```python
from build123d import *

# Parameters (mm, degrees)
BOSS_EXTRU_1_DEPTH      = 2
ESQUISSE2_R             = 1.5
ENL_V_MAT_EXTRU_1_DEPTH = 2


with BuildPart() as part:
    # Esquisse1 → Boss.-Extru.1 (new body)
    with BuildSketch(Plane.XY):
        with BuildLine():
            Line((-36.939711753, -10.835982903), (-28.105322833, -36.349774711))
            ThreePointArc((-28.105322833, -36.349774711), (-25.588682721, -38.027012465), (-23.297783694, -36.052579486))
            Line((-23.297783694, -36.052579486), (-18.763886374, -14.728100955))
            ThreePointArc((-18.763886374, -14.728100955), (-18.961021654, -12.824866099), (-20.44620762, -11.61847152))
            Line((-20.44620762, -11.61847152), (-33.863669528, -7.622008589))
            ThreePointArc((-33.863669528, -7.622008589), (-36.383421268, -8.289397427), (-36.939711753, -10.835982903))
        make_face()
        Polygon((-24.085912758, -15.751447914), (-26.31791891, -26.23061998), (-30.620361937, -13.805127209), align=None, mode=Mode.SUBTRACT)
    extrude(amount=-BOSS_EXTRU_1_DEPTH)

    # Esquisse2 → Enlèv. mat.-Extru.1 (cut)
    with BuildSketch(Plane.XY):
        with Locations((-34.577323623, -10.017983929)):
            Circle(ESQUISSE2_R)
        with Locations((-21.159861715, -14.01444686)):
            Circle(ESQUISSE2_R)
    extrude(amount=-ENL_V_MAT_EXTRU_1_DEPTH, mode=Mode.SUBTRACT)


solid = part.part
```
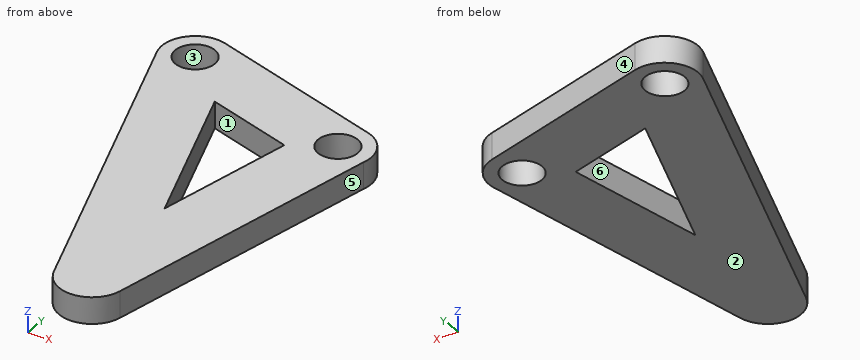
Verification items for the finished model (mm, model axes). Face numbers are marked on the shaded views. A direction names the side the tool comes from. Round coordinates to 2 decimals unless told otherwise and drop trailing zeros. Order: outer loops, then holes, each group sorted by start corner. A loop starts at its lowest first (then second) coordinate and runs counter-clockwise, first axis right, second up. Notation, with made-up numbers: (-14, -17.5) -> (9, -17.5) arc R14 ccw to (9, 6.5) -> close; hole circle Ø4 at (82.25, 47.5). An arc over 180 degrees is marked (long way). Put each result on its own line as item: value. Start each with the question number.
(1) Tool access check on the marked faces 5 and 6. Record the directions out of +Z, -Z, +X, -X, +Y, -Y that give a thin tool (end or side, any length) a straight path to the whole face; none if there is none.
(2) Section check B-B (y = -23). Enter the section's corners in (x, z), then the cut area to 3 significant figures.
(3) Draft check along Y on the marked faces 1, 2, 3 and 4. Enter one of: +Y half, -Y half, draft (parallel to the pull), parting line (faces both ways), or undercut.
(4) Section check C-C (z = -0.75). Enter the section's corners in (x, y).
(5) Section check D-D (x = -31.25). Enter the section's corners in (y, z).
(6) Section check A-A (x = -20). Enter the section's corners in (y, z), then the cut area to 3 significant figures.
(7) Depth check by flat-ended pin: pin 1 Ø1 at (y, z) = (-34, -1.5) entering from +X. Enter the tip coordinate at first touch or a pass-through.
(8) Material ranges on line 1 along X through (y, z) = (-19, -0.9); line 2 along X through (y, z) = (-25, -0.8); line 3 along X through (y, z) = (-28.5, -0.3), recorded low to high.
Completed:
1. face 5: +Z, -Z, +X, -Y
1. face 6: +Z, -Z
2. outline: (-32.73, -2) -> (-27.44, -2) -> (-27.44, 0) -> (-32.73, 0) -> close; (-25.63, -2) -> (-20.52, -2) -> (-20.52, 0) -> (-25.63, 0) -> close
2. area: 20.8 mm2
3. face 1: undercut
3. face 2: draft
3. face 3: undercut
3. face 4: +Y half
4. outline: (-36.94, -10.84) -> (-28.11, -36.35) arc R2.5 ccw to (-23.3, -36.05) -> (-18.76, -14.73) arc R2.5 ccw to (-20.45, -11.62) -> (-33.86, -7.62) arc R2.5 ccw to start; hole circle Ø3 at (-34.58, -10.02); hole (-30.62, -13.81) -> (-26.32, -26.23) -> (-24.09, -15.75) -> close; hole circle Ø3 at (-21.16, -14.01)
5. outline: (-27.27, -2) -> (-8.4, -2) -> (-8.4, 0) -> (-27.27, 0) -> close
6. outline: (-20.54, -2) -> (-14.97, -2) -> (-14.97, 0) -> (-20.54, 0) -> close; (-13.06, -2) -> (-11.8, -2) -> (-11.8, 0) -> (-13.06, 0) -> close
6. area: 13.7 mm2
7. pin 1: stops at x = -22.76
8. line 1: x = -34.11 to -28.82, -24.78 to -19.67
8. line 2: x = -32.04 to -26.74, -26.06 to -20.95
8. line 3: x = -30.82 to -21.69
